Geometry check sheet. Reference: the model listing, model coordinates, mm. Face numbers are marked on the shaded views. A direction names the side the tool comes from. Coordinates: 2 decimals unless noted, no trailing zeros. Loops run counter-clockwise (first coordinate to the right, second up) from the corner with the lowest first, then second, coordinate; pieces in that order, holes last.
from build123d import *

# Parameters (mm, degrees)
F0_W      = 100
F0_H      = 100
F1_DEPTH  = 20
F2_R      = 50
F4_DEPTH  = 10
F6_ANGLE  = 90
F7_W      = 50
F7_H      = 50
F8_DEPTH  = 10
F10_DEPTH = 60
F11_SIZE  = 5
F12_R     = 5
F16_R     = 35
F17_DEPTH = 10
F18_R     = 5


with BuildPart() as f1:
    # F0 (on Top) → F1 (new body)
    with BuildSketch(Plane.XY):
        Rectangle(F0_W, F0_H)
    extrude(amount=F1_DEPTH)

    # F2
    f2_edges = [f1.edges().sort_by_distance(p)[0] for p in [
        (50, 50, 10),
    ]]
    fillet(f2_edges, radius=F2_R)

    # F3 (on face) → F4 (cut)
    with BuildSketch(Plane.XY.offset(20)):
        with BuildLine():
            ThreePointArc((50, 0), (35.3553390593, -35.3553390593), (0, -50))
            Line((0, -50), (50, -50))
            Line((50, -50), (50, 0))
        make_face()
    extrude(amount=-F4_DEPTH, mode=Mode.SUBTRACT)

    # F5 (on Front) → F6 (revolve)
    with BuildSketch(Plane.XZ):
        with BuildLine():
            ThreePointArc((0, 70), (-35.3553390593, 55.3553390593), (-50, 20))
            Line((-50, 20), (0, 20))
            Line((0, 20), (0, 70))
        make_face()
    revolve(axis=Axis((0, 0, 45), (0, 0, 1)), revolution_arc=F6_ANGLE)

    # F7 (on face) → F8 (cut)
    with BuildSketch(Plane.XY.offset(20)):
        with Locations((-25, 25)):
            Rectangle(F7_W, F7_H)
    extrude(amount=-F8_DEPTH, mode=Mode.SUBTRACT)

    # F9 (on face) → F10 (join)
    with BuildSketch(Plane.XY.offset(10)):
        with BuildLine():
            ThreePointArc((0, 50), (-35.3553390593, 35.3553390593), (-50, 0))
            Line((-50, 0), (0, 0))
            Line((0, 0), (0, 50))
        make_face()
    extrude(amount=F10_DEPTH)

    # F11
    f11_edges = [f1.edges().sort_by_distance(p)[0] for p in [
        (-35.355339, 35.355339, 70),
    ]]
    chamfer(f11_edges, length=F11_SIZE)

    # F12
    f12_edges = [f1.edges().sort_by_distance(p)[0] for p in [
        (-50, 50, 5),
        (50, -50, 5),
    ]]
    fillet(f12_edges, radius=F12_R)

    # F13 (on face) → F15 section 0
    with BuildSketch(Plane.XY.offset(20), mode=Mode.PRIVATE) as f15_s0:
        Polygon((50, 0), (0, 50), (0, 0), align=None)
    loft([f15_s0.sketch, Vertex(0, 0, 70)])

    # F16 (on face) → F17 (cut)
    with BuildSketch(Plane(origin=(0, 0, 0), x_dir=(1, 0, 0), z_dir=(0, 0, -1))):
        Circle(F16_R)
    extrude(amount=-F17_DEPTH, mode=Mode.SUBTRACT)

    # F18
    f18_edges = [f1.edges().sort_by_distance(p)[0] for p in [
        (-35, 0, 10),
    ]]
    fillet(f18_edges, radius=F18_R)


solid = f1.part
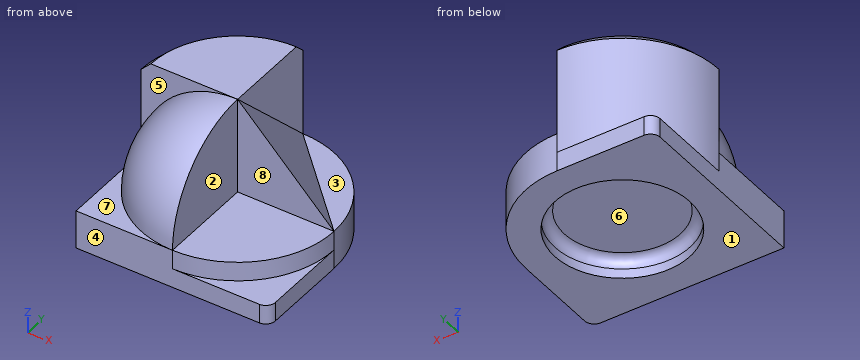
(1) Draft check along Y on the marked faces 6, 7 and 8. Enter one of: +Y half, -Y half, draft (parallel to the pull), parting line (faces both ways), or undercut.
Findings:
face 6: undercut
face 7: draft
face 8: -Y half
(2) Sectioned sample at B-B on z = 59. Record the cut outline in (x, y), and give its area (3 significant figures).
Findings:
outline: (-50, 0) - (-31.29, 0) arc R31.29 ccw to (0, -31.29) - (0, 0) - (11, 0) - (0, 11) - (0, 50) arc R50 ccw to start
area: 2,790 mm2
(3) Scan lines: L1, parallel to Y at x = 0, z = 1; L2, parallel to Z at x = -34.5, y = 44. Record each from-to range of solid material in increasing order.
Findings:
L1: y = -50 to -35, 35 to 50
L2: z = 0 to 10
(4) Sectioned sample at C-C on z = 44.5. Record the cut outline in (x, y).
Findings:
outline: (-50, 0) - (-43.59, 0) arc R43.59 ccw to (0, -43.59) - (0, 0) - (25.5, 0) - (0, 25.5) - (0, 50) arc R50 ccw to start
(5) Sectioned sample at A-A on y = -40. Record the cut outline in (x, z), and give its area (3 significant figures).
Findings:
outline: (-50, 0) - (50, 0) - (50, 10) - (30, 10) - (30, 20) - (0, 20) - (0, 50) arc R30 ccw to (-30, 20) - (-50, 20) - close
area: 2,510 mm2
(6) Gauge pin test, flat ends, axial feed: pin 1 Ø25 at (x, y) = (-25, -20.5) entering from +Z; pin 2 Ø15 at (x, y) = (28.5, 24.5) entering from +Z; pin 3 Ø5 at (x, z) = (-6.5, 23.5) entering from -Y. Record the tip position at first contact, or that the pin passes through.
Findings:
pin 1: stops at z = 65.9
pin 2: stops at z = 27.61
pin 3: stops at y = -49.76
(7) Access from +Z, -Z, +X, -X, +Y, -Y to the whole of each face (thin tool, end or side, straight path). Record for the marked faces 1, 2, 3, 4 and 5.
Findings:
face 1: -Z, +X, -X, +Y, -Y
face 2: +Z, +X, -Y
face 3: +Z, +X, +Y
face 4: +Z, -Z, +X, -X, -Y
face 5: +Z, -X, -Y
